The figure shows three views and two pictorial views of one solid part (mm, origin at its lowest corner). Answer the questions. A direction names the side the tool comes from. Coordinates: 2 decimals unless noted, no trailing zeros. Order: outer loops, then holes, each group sorted by start corner. A loop starts at its lowest first (then second) coordinate and runs counter-clockwise, first axis right, second up. Notation, with made-up numbers: (-7, -14.5) - (41, -14.5) arc R17 cw to (41, -10.5) - close; hole circle Ø11 at (-24, 89). An arc over 180 degrees is marked (long way). Use one line per item in the form item = value. Start each with the question number.
Item 1: A tool of negligible diameter and unlimited length cuts with its end or side. For the marked faces 5 and 6, from which of +Z, -Z, +X, -X, +Y, -Y can it reach the whole face along a straight path? Write none if from no direction.
Item 2: Consider line 1 along X through (y, z) = (5.25, 8.25); line 2 along Y through (x, z) = (4, 1.3); line 3 along Z through (x, y) = (37.5, 6.25). Determine where each line is inside the solid, lowest interval first. Write a range as [from, to].
Item 3: Section C-C, the plane z = 3.5 is taken. Write down the section's boundary in (x, y).
Item 4: Each of these flat-tipped pins is pushed along its axis until it touches: pin 1 Ø5 at (x, y) = (21.5, 5.5) entering from +Z; pin 2 Ø5 at (y, z) = (5, 1.5) entering from -X; pin 3 Ø1.5 at (y, z) = (8, 6) entering from +X. Where does it stop, or does it pass through?
Item 5: The mould has two halves that part along Y. Classify the marked faces 1, 2, 3 and 4: released by +Y, released by -Y, zero draft, split by the parting line, or undercut.
Item 6: Section B-B, the plane x = 46 is taken. Write down the section's boundary in (y, z), and give its area (3 significant figures).
Item 7: Section D-D, the plane x = 4 is taken. Write down the section's boundary in (y, z).
Item 8: Section A-A, the plane y = 5 is taken. Write down the section's boundary in (x, z).
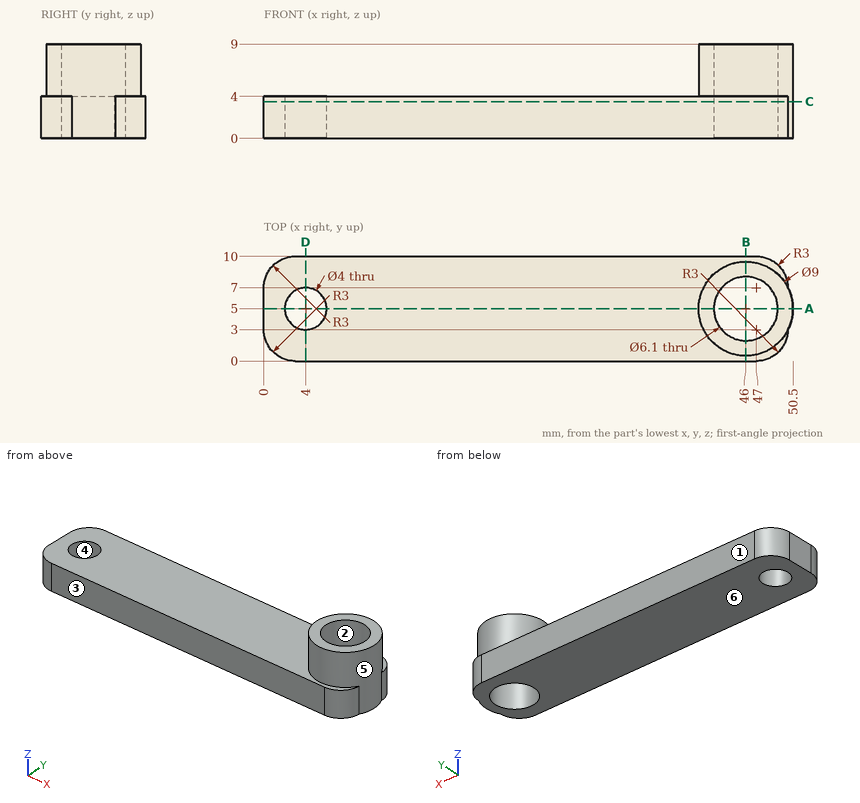
Response:
q1.face_5 = +Z
q1.face_6 = -Z, +X, -X, +Y, -Y
q2.line_1 = [41.51, 42.96], [49.04, 50.49]
q2.line_2 = [0, 3], [7, 10]
q2.line_3 = [0, 4]
q3.outline = (0, 3) arc R3 ccw to (3, 0) - (47, 0) arc R3 ccw to (50, 2.94) arc R4.5 ccw to (50, 7.06) arc R3 ccw to (47, 10) - (3, 10) arc R3 ccw to (0, 7) - close; hole circle Ø4 at (4, 5); hole circle Ø6.1 at (46, 5)
q4.pin_1 = 4
q4.pin_2 = 0
q4.pin_3 = 49.9
q5.face_1 = released by +Y
q5.face_2 = undercut
q5.face_3 = released by -Y
q5.face_4 = undercut
q6.outline = (0, 0) - (1.95, 0) - (1.95, 9) - (0.5, 9) - (0.5, 4) - (0, 4) - close; (8.05, 0) - (10, 0) - (10, 4) - (9.5, 4) - (9.5, 9) - (8.05, 9) - close
q6.area = 30.1 mm2
q7.outline = (0, 0) - (3, 0) - (3, 4) - (0, 4) - close; (7, 0) - (10, 0) - (10, 4) - (7, 4) - close
q8.outline = (0, 0) - (2, 0) - (2, 4) - (0, 4) - close; (6, 0) - (42.95, 0) - (42.95, 9) - (41.5, 9) - (41.5, 4) - (6, 4) - close; (49.05, 0) - (50.5, 0) - (50.5, 9) - (49.05, 9) - close
